Read the model definition and answer for the solid it produces. Units are mm, in the model's axes. A direction names the side the tool comes from. Coordinates: 2 decimals unless noted, no trailing zeros. Write each loop counter-clockwise with the first axis right and the second up, starting at its lowest first coordinate (ties: lowest second). Pieces come first, ordered by that corner, then holes.
(1) The part is cut by section A-A, the plane z = 15.25. Determine the outline of the cut face in (x, y), and give its area (3 significant figures).
(2) Determine the mould class of faces 1 (the flat face through (-17, -11, 16.5)), 2 (the flat face through (-17, -17.953, 16)), 3 (the flat face through (-17, -19.523, 8)) for opening direction Y: pulls with the +Y half, pulls with the -Y half, needs draft (parallel to the pull), parting line crosses it, or undercut.
(3) The part is cut by section D-D, the plane z = 2.5. Determine the outline of the cut face in (x, y), and give its area (3 significant figures).
(4) Straight lines are drawn through the part: line 1 along Y through (x, z) = (-19, 6.25); line 2 along X through (y, z) = (-7.75, 6.5); line 3 along Z through (x, y) = (-13.5, -13). For each, find the intervals that lie inside material, in ascending order.
(5) Given pin 1 (4 mm diameter, centred on y = -9, z = 9, fed in from -X), flat-ended and moving along its own axis, determine where the tip first touches the part or whether it passes through.
(6) The part is cut by section C-C, the plane y = -16. Determine the outline of the cut face in (x, z).
(7) Which of the six approach directions +Z, -Z, +X, -X, +Y, -Y give full straight-line access (tool end or side, diameter ignored) to faces 4 (the flat face through (-17, -12.076, 16)), 5 (the flat face through (-18, -8, 12)), 6 (the flat face through (-17, -8, 16.5))?
```python
from build123d import *

# Parameters (mm, degrees)
F0_W     = 5.5
F0_H     = 16.3
F0_W_2   = 2.3349355608
F0_H_2   = 2.2036070004
F1_DEPTH = 15
F2_DEPTH = 12
F3_W     = 10.8860824257
F3_H     = 1.5700478107
F3_H_2   = 1.4735469595
F3_H_3   = 1.5152581036
F3_H_4   = 1.5589032643
F3_H_5   = 1.1953348294
F3_H_6   = 1.0883370414
F3_H_7   = 1.4443685184
F4_DEPTH = 1.5


with BuildPart() as f1:
    # F0 (on Top) → F1 (new body)
    with BuildSketch(Plane.XY):
        with Locations((-19.2246585935, -7.1874150395)):
            Rectangle(F0_W, F0_H)
        Polygon((-14.1397230327, 0.9625849605), (-16.4746585935, 0.9625849605), (-16.4746585935, -15.3374150395), (-16.4746585935, -15.3418527916), (-14.1397230327, -15.3418527916), align=None)
        Polygon((-16.4746585935, -15.3374150395), (-21.9746585935, -15.3374150395), (-21.9746585935, -17.545459792), (-16.4746585935, -17.545459792), (-16.4746585935, -15.3418527916), align=None)
        Polygon((-11.0885761678, 0.9625849605), (-14.1397230327, 0.9625849605), (-14.1397230327, -15.3418527916), (-14.1397230327, -17.545459792), (-11.0885761678, -17.545459792), align=None)
        Polygon((-16.4746585935, -17.545459792), (-21.9746585935, -17.545459792), (-21.9746585935, -19.5230543613), (-11.0885761678, -19.5230543613), (-11.0885761678, -17.545459792), (-14.1397230327, -17.545459792), align=None)
        with Locations((-15.3071908131, -16.4436562918)):
            Rectangle(F0_W_2, F0_H_2)
    extrude(amount=F1_DEPTH)

    # F0 (on Top) → F2 (cut)
    with BuildSketch(Plane.XY):
        Polygon((-14.1397230327, 0.9625849605), (-16.4746585935, 0.9625849605), (-16.4746585935, -15.3374150395), (-16.4746585935, -15.3418527916), (-14.1397230327, -15.3418527916), align=None)
        with Locations((-19.2246585935, -7.1874150395)):
            Rectangle(F0_W, F0_H)
        Polygon((-16.4746585935, -15.3374150395), (-21.9746585935, -15.3374150395), (-21.9746585935, -17.545459792), (-16.4746585935, -17.545459792), (-16.4746585935, -15.3418527916), align=None)
        with Locations((-15.3071908131, -16.4436562918)):
            Rectangle(F0_W_2, F0_H_2)
    extrude(amount=F2_DEPTH, mode=Mode.SUBTRACT)

    # F3 (on face) → F4 (join)
    with BuildSketch(Plane.XY.offset(15)):
        with Locations((-16.5316173807, -18.738030456)):
            Rectangle(F3_W, F3_H)
        with Locations((-16.5316173807, -14.8630174808)):
            Rectangle(F3_W, F3_H_2)
        with Locations((-16.5316173807, -11.318010278)):
            Rectangle(F3_W, F3_H_3)
        with Locations((-16.5316173807, -8.5007830683)):
            Rectangle(F3_W, F3_H_4)
        with Locations((-16.5316173807, -5.3385491483)):
            Rectangle(F3_W, F3_H_5)
        with Locations((-16.5316173807, -2.6988773607)):
            Rectangle(F3_W, F3_H_6)
        with Locations((-16.5316173807, 0.2404007013)):
            Rectangle(F3_W, F3_H_7)
    extrude(amount=F4_DEPTH)


solid = f1.part
```
Computed:
1. outline: (-21.97, -19.52) - (-11.09, -19.52) - (-11.09, -17.95) - (-21.97, -17.95) - close; (-21.97, -15.6) - (-11.09, -15.6) - (-11.09, -14.13) - (-21.97, -14.13) - close; (-21.97, -12.08) - (-11.09, -12.08) - (-11.09, -10.56) - (-21.97, -10.56) - close; (-21.97, -9.28) - (-11.09, -9.28) - (-11.09, -7.72) - (-21.97, -7.72) - close; (-21.97, -5.94) - (-11.09, -5.94) - (-11.09, -4.74) - (-21.97, -4.74) - close; (-21.97, -3.24) - (-11.09, -3.24) - (-11.09, -2.15) - (-21.97, -2.15) - close; (-21.97, -0.48) - (-11.09, -0.48) - (-11.09, 0.96) - (-21.97, 0.96) - close
1. area: 107 mm2
2. face 1: needs draft
2. face 2: undercut
2. face 3: pulls with the -Y half
3. outline: (-21.97, -19.52) - (-11.09, -19.52) - (-11.09, 0.96) - (-14.14, 0.96) - (-14.14, -17.55) - (-21.97, -17.55) - close
3. area: 78.0 mm2
4. line 1: y = -19.52 to -17.55
4. line 2: x = -14.14 to -11.09
4. line 3: z = 0 to 15
5. pin 1: stops at x = -14.14
6. outline: (-21.97, 12) - (-14.14, 12) - (-14.14, 0) - (-11.09, 0) - (-11.09, 15) - (-21.97, 15) - close
7. face 4: +Z, +X, -X
7. face 5: -Z, -X, +Y
7. face 6: +Z, +X, -X, +Y, -Y
